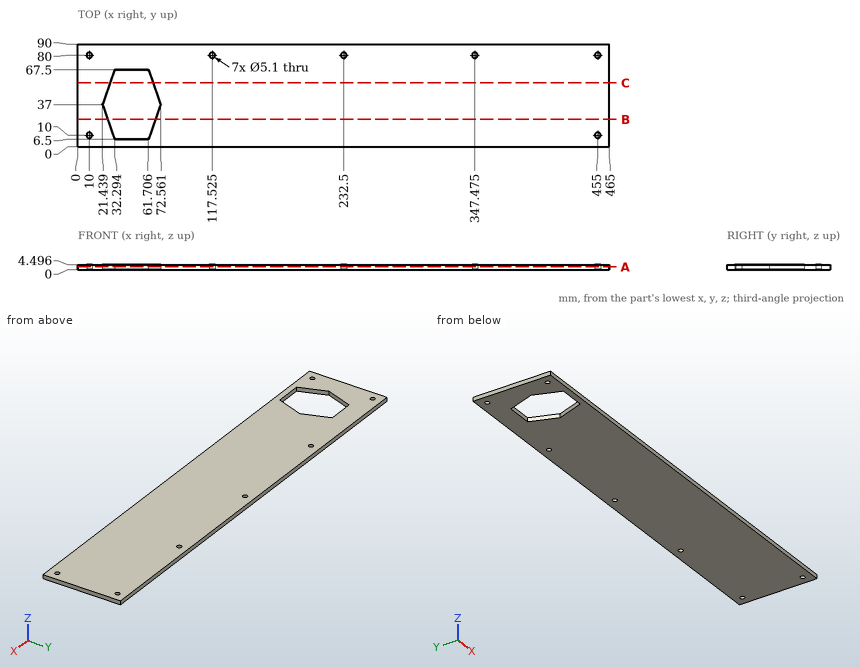
Geometry check sheet. Reference: drawing and pictorial views, mm from the part's lowest x, y, z. Give positions to 0.01 mm unless a question says otherwise; leave off trailing zeros. Write each loop counter-clockwise with the first axis right and the second up, starting at its lowest first coordinate (ties: lowest second). Pieces come first, ordered by that corner, then holes. Notation, with made-up numbers: M 46,18 L 70,18 A26 cw 70,53 Z; hole C 67,38 d11. An arc over 180 degrees is marked long. Put each result on its own line as item: value. Start each with the question number.
1. Section check B-B (y = 24). Record the cut outline in (x, z) (1 decimal), and give its area (3 significant figures).
2. Section check A-A (z = 2.6). Give the number of separate pieces and of enclosed holes in the cut face, and give its area (4 significant figures).
3. Section check C-C (y = 56). Record the cut outline in (x, z) (1 decimal).
4. Scan lines: line 1 along Y through (x, z) = (455, 1.2); line 2 along Y through (x, z) = (232.5, 1.4); line 3 along X through (y, z) = (8.5, 2.7) (1 decimal). Record each from-to range of solid material in increasing order. Write a range as [from, to].
Answer list:
1. outline: M 0,0 L 26.1,0 L 26.1,4.5 L 0,4.5 Z; M 67.9,0 L 465,0 L 465,4.5 L 67.9,4.5 Z
1. area: 1,900 mm2
2. separate pieces: 1
2. enclosed holes: 8
2. area: 39,250 mm2
3. outline: M 0,0 L 28.2,0 L 28.2,4.5 L 0,4.5 Z; M 65.8,0 L 465,0 L 465,4.5 L 65.8,4.5 Z
4. line 1: [0, 7.45], [12.55, 77.45], [82.55, 90]
4. line 2: [0, 77.45], [82.55, 90]
4. line 3: [0, 7.9], [12.1, 31.6], [62.4, 452.9], [457.1, 465]
